Build history of the part. All positions in model axes, mm. Round coordinates to 2 decimals unless told otherwise and drop trailing zeros. Order: outer loops, then holes, each group sorted by start corner. A loop starts at its lowest first (then second) coordinate and runs counter-clockwise, first axis right, second up. Notation, with made-up numbers: (73, 22.5) -> (129, 22.5) arc R22 cw to (129, 59.5) -> close; hole circle Ø3 at (-27.5, -39). An arc over 180 degrees is marked (long way). Answer as a JSON object with one key per item and string values.
from build123d import *

# Parameters (mm, degrees)
F0_W      = 740
F0_H      = 200
F1_DEPTH  = 9
F2_W      = 4.5
F2_H      = 200
F3_DEPTH  = 4.5
F4_W      = 4.5
F4_H      = 200
F5_DEPTH  = 4.5
F6_W      = 731
F6_H      = 4.5
F7_DEPTH  = 4.5
F8_W      = 150
F8_H      = 31
F9_DEPTH  = 9
F10_W     = 148
F10_H     = 42.5
F11_DEPTH = 9.001
F12_W     = 4.5
F12_H     = 45
F13_DEPTH = 4.5
F14_W     = 9
F14_H     = 200
F15_DEPTH = 20
F16_W     = 9
F16_H     = 200
F17_DEPTH = 20


with BuildPart() as f1:
    # F0 (on Front) → F1 (new body)
    with BuildSketch(Plane.XZ):
        Rectangle(F0_W, F0_H)
    extrude(amount=F1_DEPTH)

    # F2 (on face) → F3 (cut)
    with BuildSketch(Plane.YZ.offset(370)):
        with Locations((-2.25, 0)):
            Rectangle(F2_W, F2_H)
    extrude(amount=-F3_DEPTH, mode=Mode.SUBTRACT)

    # F4 (on face) → F5 (cut)
    with BuildSketch(Plane(origin=(-370, 0, 0), x_dir=(0, -1, 0), z_dir=(-1, 0, 0))):
        with Locations((2.25, 0)):
            Rectangle(F4_W, F4_H)
    extrude(amount=-F5_DEPTH, mode=Mode.SUBTRACT)

    # F6 (on face) → F7 (cut)
    with BuildSketch(Plane(origin=(0, 0, 0), x_dir=(-1, 0, 0), z_dir=(0, 1, 0))):
        with Locations((0, -52.75)):
            Rectangle(F6_W, F6_H)
    extrude(amount=-F7_DEPTH, mode=Mode.SUBTRACT)

    # F8 (on face) → F9 (cut, through all)
    with BuildSketch(Plane.XZ.offset(9)):
        with Locations((270, -79.5)):
            Rectangle(F8_W, F8_H)
    extrude(amount=-F9_DEPTH, mode=Mode.SUBTRACT)

    # F10 (on face) → F11 (cut, through all)
    with BuildSketch(Plane(origin=(0, 0, 0), x_dir=(-1, 0, 0), z_dir=(0, 1, 0))):
        with Locations((-39.5, -78.75)):
            Rectangle(F10_W, F10_H)
    extrude(amount=-F11_DEPTH, mode=Mode.SUBTRACT)

    # F12 (on face) → F13 (cut)
    with BuildSketch(Plane(origin=(0, 0, 0), x_dir=(-1, 0, 0), z_dir=(0, 1, 0))):
        with Locations((36.75, -77.5)):
            Rectangle(F12_W, F12_H)
        with Locations((-115.75, -77.5)):
            Rectangle(F12_W, F12_H)
    extrude(amount=-F13_DEPTH, mode=Mode.SUBTRACT)

    # F14 (on face) → F15 (join)
    with BuildSketch(Plane.YZ.offset(370)):
        with Locations((-4.5, 0)):
            Rectangle(F14_W, F14_H)
    extrude(amount=F15_DEPTH)

    # F16 (on face) → F17 (join)
    with BuildSketch(Plane(origin=(-370, 0, 0), x_dir=(0, -1, 0), z_dir=(-1, 0, 0))):
        with Locations((4.5, 0)):
            Rectangle(F16_W, F16_H)
    extrude(amount=F17_DEPTH)


solid = f1.part
1) Probe L1, parallel to X at y = -1.5, z = -20; L2, parallel to X at y = -3, z = -75; L3, parallel to X at y = -5, z = -70. List the from-to ranges inside material, lowest first. Write a range as from..to.
Checked values:
{"L1": "x = -390..-370, -365.5..365.5, 370..390", "L2": "x = -390..-370, -365.5..-39, 118..195, 345..365.5, 370..390", "L3": "x = -390..-34.5, 113.5..195, 345..390"}
2) Pull direction X, two halves, no side cores. Call faces 1 (the face through (5, -9, -1)), 2 (the face through (-2, -4.5, -52)): pulls with the +X half, pulls with the -X half, needs draft (parallel to the pull), parting line crosses it, or undercut.
Checked values:
{"face 1": "needs draft", "face 2": "undercut"}
3) Flat gauge pin, fed straight in: pin 1 Ø3 at (x, z) = (239, 0) entering from +Y. Where does the tip first touch, or does it go through?
Checked values:
{"pin 1": "stops at y = 0"}
4) Cut at A-A, the plane y = -1.75. Give the cut face in (x, z).
Checked values:
{"outline": "(-390, -100) -> (-370, -100) -> (-370, 100) -> (-390, 100) -> close; (-365.5, -100) -> (-39, -100) -> (-39, -55) -> (-365.5, -55) -> close; (-365.5, -50.5) -> (365.5, -50.5) -> (365.5, 100) -> (-365.5, 100) -> close; (-34.5, -57.5) -> (113.5, -57.5) -> (113.5, -55) -> (-34.5, -55) -> close; (118, -100) -> (365.5, -100) -> (365.5, -55) -> (118, -55) -> close; (370, -100) -> (390, -100) -> (390, 100) -> (370, 100) -> close; hole (195, -95) -> (345, -95) -> (345, -64) -> (195, -64) -> close"}
5) Cut at B-B, the plane x = 255.5. Give the cut face in (y, z), plus the area to 3 significant figures.
Checked values:
{"outline": "(-9, -100) -> (0, -100) -> (0, -95) -> (-9, -95) -> close; (-9, -64) -> (0, -64) -> (0, -55) -> (-4.5, -55) -> (-4.5, -50.5) -> (0, -50.5) -> (0, 100) -> (-9, 100) -> close", "area": "1,500 mm²"}
6) Cut at C-C, the plane x = 33. Give the cut face in (y, z), plus the area to 3 significant figures.
Checked values:
{"outline": "(-9, -57.5) -> (0, -57.5) -> (0, -55) -> (-4.5, -55) -> (-4.5, -50.5) -> (0, -50.5) -> (0, 100) -> (-9, 100) -> close", "area": "1,400 mm²"}
